Here's how the part is built. I have some questions about the finished solid (model axes, mm). Coordinates: 2 decimals unless noted, no trailing zeros. Write each loop counter-clockwise with the first axis right and the second up, starting at its lowest first coordinate (ties: lowest second). Pieces come first, ordered by that corner, then holes.
(1) Please list where these lines run through material, in increasing order: probe 1 along Y at (x, z) = (0, 2.9); probe 2 along Y at (x, z) = (-25.4, 1.1); probe 3 along Y at (x, z) = (30, 0.2).
(2) Imagine slicing it at B-B, the plane y = -56.65. List the corners of the cut face in (x, z) for me.
(3) Imagine slicing it at C-C, the plane z = 1.2. List the corners of the cut face in (x, y) for me, plus the area to 3 significant figures.
(4) Imagine slicing it at D-D, the plane y = -95.25. List the corners of the cut face in (x, z) for me, plus the area to 3 significant figures.
(5) Imagine slicing it at A-A, the plane x = 0. List the corners of the cut face in (y, z) for me, plus the area to 3 significant figures.
Autodesk Inventor part; units mm, degrees
ref_plane "Work Plane1" through (0, -135.7786, 0) normal (0, 0, 1) x (1, 0, 0)
ref_plane "YZ Plane" through (0, 0, 0) normal (1, 0, 0) x (0, 1, 0)
ref_plane "XZ Plane" through (0, 0, 0) normal (0, 1, 0) x (-1, 0, 0)
sketch "Sketch1" plane through (0, 0, 0) normal (0, 0, 1) x (1, 0, 0)
  line L0 (6.35, -214.55) -> (43.1, -214.55)
  line L1 (43.1, -214.55) -> (43.1, -189.15)
  line L2 (43.1, -189.15) -> (40.1028, -189.15)
  line L3 (40.1028, -189.15) -> (40.1028, -176.45)
  line L4 (40.1028, -176.45) -> (43.1, -176.45)
  line L5 (43.1, -176.45) -> (43.1, -110.25)
  line L6 (43.1, -110.25) -> (40.1028, -110.25)
  line L7 (40.1028, -110.25) -> (40.1028, -97.55)
  line L8 (40.1028, -97.55) -> (43.1, -97.55)
  line L9 (43.1, -97.55) -> (43.1, -72.15)
  line L10 (43.1, -72.15) -> (35.023, -72.15)
  arc A0 (-35.023, -72.15) -> (35.023, -72.15) centre (0, -57.15) ccw
  line L11 (-35.023, -72.15) -> (-43.1, -72.15)
  line L12 (-43.1, -72.15) -> (-43.1, -97.55)
  line L13 (-43.1, -97.55) -> (-40.1028, -97.55)
  line L14 (-40.1028, -97.55) -> (-40.1028, -110.25)
  line L15 (-40.1028, -110.25) -> (-43.1, -110.25)
  line L16 (-43.1, -110.25) -> (-43.1, -176.45)
  line L17 (-43.1, -176.45) -> (-40.1028, -176.45)
  line L18 (-40.1028, -176.45) -> (-40.1028, -189.15)
  line L19 (-40.1028, -189.15) -> (-43.1, -189.15)
  line L20 (-43.1, -189.15) -> (-43.1, -214.55)
  line L21 (-43.1, -214.55) -> (-6.35, -214.55)
  line L22 (-11.16, -143.04) -> (-11.16, -138.135)
  line L23 (-11.16, -138.135) -> (10.16, -138.135)
  line L24 (10.16, -138.135) -> (10.16, -168.265)
  line L25 (10.16, -168.265) -> (-11.16, -168.265)
  line L26 (-11.16, -168.265) -> (-11.16, -159.55)
  line L27 (-11.16, -159.55) -> (-19.058, -159.55)
  line L28 (-19.058, -159.55) -> (-19.058, -164.622)
  line L29 (-19.058, -164.622) -> (-22.598, -164.622)
  line L30 (-22.598, -164.622) -> (-22.598, -159.55)
  line L31 (-22.598, -159.55) -> (-32.258, -159.55)
  line L32 (-32.258, -159.55) -> (-32.258, -167.805)
  line L33 (-32.258, -167.805) -> (-34.29, -167.805)
  line L34 (-34.29, -167.805) -> (-34.29, -159.55)
  line L35 (-34.29, -159.55) -> (-38.1, -159.55)
  line L36 (-38.1, -159.55) -> (-38.1, -136.69)
  line L37 (-38.1, -136.69) -> (-22.598, -136.69)
  line L38 (-22.598, -136.69) -> (-22.598, -131.618)
  line L39 (-22.598, -131.618) -> (-19.058, -131.618)
  line L40 (-19.058, -131.618) -> (-19.058, -136.69)
  line L41 (-19.058, -136.69) -> (-15.24, -136.69)
  line L42 (-15.24, -136.69) -> (-15.24, -143.04)
  arc A1 (-38.1, -57.15) -> (38.1, -57.15) centre (0, -57.15) ccw
  line L43 (0, -57.15) -> (0, -82.55)
  circle A2 centre (0, -82.55) radius 38.1
  line L44 (38.1, -82.55) -> (-38.1, -82.55)
  line L45 (-38.1, -82.55) -> (-38.1, -44.45)
  line L46 (-38.1, -44.45) -> (38.1, -44.45)
  line L47 (38.1, -44.45) -> (38.1, -82.55)
  circle A3 centre (25.4, -95.25) radius 1.5
  circle A4 centre (-25.4, -95.25) radius 1.5
  line L48 (-15.24, -143.04) -> (-11.16, -143.04)
  line L49 (-6.35, -214.55) -> (-6.35, -203.8154)
  line L50 (-6.35, -203.8154) -> (6.35, -203.8154)
  line L51 (6.35, -203.8154) -> (6.35, -214.55)
  point P0 (0, 0)
  dimension "d1" = 76.2
  dimension "d0" = 25.4
extrude "Extrusion1" add sketch "Sketch1" along normal blind 4 contours L47 A2 L10 | L10 A2 A1 L47 | A2 L44 A0 L10 | L10 A1 A2 | A1 A2 L46 L47 | A2 L44 A0 | A0 L44 A1 A2 | L45 L11 A2 | A2 L11 A0 L44 | A0 L44 | A2 A1 L45 L46 | A2 A1 L11 | L11 L45 A1 A2 | A3 | A4
ref_plane "Work Plane1" through (0, -135.7786, 0) normal (0, 0, 1) x (1, 0, 0)
sketch "Sketch2" plane through (0, 0, 4) normal (0, 0, 1) x (1, 0, 0)
  line L0 (-40.1, -31.75) -> (-43.1, -31.75)
  line L1 (-43.1, -31.75) -> (-43.1, -57.15)
  line L2 (-43.1, -57.15) -> (-38.1, -57.15)
  arc A0 (-38.1, -57.15) -> (38.1, -57.15) centre (0, -57.15) ccw
  line L3 (38.1, -57.15) -> (43.1, -57.15)
  line L4 (43.1, -57.15) -> (43.1, -31.75)
  line L5 (43.1, -31.75) -> (40.1, -31.75)
  line L6 (40.1, -31.75) -> (40.1, -19.05)
  line L7 (40.1, -19.05) -> (43.1, -19.05)
  line L8 (43.1, -19.05) -> (43.1, 24.05)
  line L9 (43.1, 24.05) -> (40.1, 24.05)
  line L10 (40.1, 24.05) -> (40.1, 36.75)
  line L11 (40.1, 36.75) -> (43.1, 36.75)
  line L12 (43.1, 36.75) -> (43.1, 62.15)
  line L13 (14, 62.15) -> (-14, 62.15)
  line L14 (-43.1, 62.15) -> (-43.1, 36.75)
  line L15 (-43.1, 36.75) -> (-40.1, 36.75)
  line L16 (-40.1, 36.75) -> (-40.1, 24.05)
  line L17 (-40.1, 24.05) -> (-43.1, 24.05)
  line L18 (-43.1, 24.05) -> (-43.1, -19.05)
  line L19 (-43.1, -19.05) -> (-40.1, -19.05)
  line L20 (-40.1, -19.05) -> (-40.1, -31.75)
  line L21 (15.24, -5.55) -> (11.16, -5.55)
  line L22 (11.16, -5.55) -> (11.16, -14.265)
  line L23 (11.16, -14.265) -> (-10.16, -14.265)
  line L24 (-10.16, -14.265) -> (-10.16, 15.865)
  line L25 (-10.16, 15.865) -> (11.16, 15.865)
  line L26 (11.16, 15.865) -> (11.16, 7.15)
  line L27 (11.16, 7.15) -> (19.058, 7.15)
  line L28 (22.598, 7.15) -> (32.266, 7.15)
  line L29 (32.266, 7.15) -> (32.266, 15.405)
  line L30 (32.266, 15.405) -> (34.282, 15.405)
  line L31 (34.282, 15.405) -> (34.282, 7.15)
  line L32 (34.282, 7.15) -> (38.1, 7.15)
  line L33 (38.1, 7.15) -> (38.1, -15.71)
  line L34 (38.1, -15.71) -> (22.598, -15.71)
  line L35 (19.058, -15.71) -> (15.24, -15.71)
  line L36 (15.24, -15.71) -> (15.24, -5.55)
  line L37 (19.058, 7.15) -> (19.058, 12.222)
  line L38 (19.058, 12.222) -> (22.598, 12.222)
  line L39 (22.598, 12.222) -> (22.598, 7.15)
  line L40 (22.598, -15.71) -> (22.598, -20.782)
  line L41 (22.598, -20.782) -> (19.058, -20.782)
  line L42 (19.058, -20.782) -> (19.058, -15.71)
  line L43 (-14, 62.15) -> (-14, 31.5)
  line L44 (-14, 31.5) -> (-30.4, 31.5)
  line L45 (-30.4, 31.5) -> (-30.4, 62.15)
  line L46 (-30.4, 62.15) -> (-43.1, 62.15)
  line L47 (43.1, 62.15) -> (30.4, 62.15)
  line L48 (30.4, 62.15) -> (30.4, 31.5)
  line L49 (30.4, 31.5) -> (14, 31.5)
  line L50 (14, 31.5) -> (14, 62.15)
  line L51 (0, -57.15) -> (0, -56.65)
  circle A1 centre (0, -56.65) radius 2.5019
  point P0 (0, 0)
  dimension "d13" = 0.5
  dimension "d14" = 5.0038
extrude "Extrusion2" cut sketch "Sketch2" against normal blind 4 contours A1
sketch "Sketch3" plane through (0, 0, 4) normal (0, 0, 1) x (1, 0, 0)
  arc A0 (-35.023, -72.15) -> (35.023, -72.15) centre (0, -57.15) ccw
  line L0 (-6.35, -214.55) -> (-6.35, -203.8154)
  line L1 (-6.35, -203.8154) -> (6.35, -203.8154)
  line L2 (6.35, -203.8154) -> (6.35, -214.55)
  line L3 (6.35, -214.55) -> (43.1, -214.55)
  line L4 (43.1, -214.55) -> (43.1, -189.15)
  line L5 (43.1, -189.15) -> (40.1028, -189.15)
  line L6 (40.1028, -189.15) -> (40.1028, -176.45)
  line L7 (40.1028, -176.45) -> (43.1, -176.45)
  line L8 (43.1, -176.45) -> (43.1, -110.25)
  line L9 (43.1, -110.25) -> (40.1028, -110.25)
  line L10 (40.1028, -110.25) -> (40.1028, -97.55)
  line L11 (40.1028, -97.55) -> (43.1, -97.55)
  line L12 (43.1, -97.55) -> (43.1, -72.15)
  line L13 (43.1, -72.15) -> (35.023, -72.15)
  arc A1 (-35.023, -72.15) -> (35.023, -72.15) centre (0, -57.15) ccw
  line L14 (-35.023, -72.15) -> (-43.1, -72.15)
  line L15 (-43.1, -72.15) -> (-43.1, -97.55)
  line L16 (-43.1, -97.55) -> (-40.1028, -97.55)
  line L17 (-40.1028, -97.55) -> (-40.1028, -110.25)
  line L18 (-40.1028, -110.25) -> (-43.1, -110.25)
  line L19 (-43.1, -110.25) -> (-43.1, -176.45)
  line L20 (-43.1, -176.45) -> (-40.1028, -176.45)
  line L21 (-40.1028, -176.45) -> (-40.1028, -189.15)
  line L22 (-40.1028, -189.15) -> (-43.1, -189.15)
  line L23 (-43.1, -189.15) -> (-43.1, -214.55)
  line L24 (-43.1, -214.55) -> (-6.35, -214.55)
  line L25 (-11.16, -143.04) -> (-11.16, -138.135)
  line L26 (-11.16, -138.135) -> (10.16, -138.135)
  line L27 (10.16, -138.135) -> (10.16, -168.265)
  line L28 (10.16, -168.265) -> (-11.16, -168.265)
  line L29 (-11.16, -168.265) -> (-11.16, -159.55)
  line L30 (-11.16, -159.55) -> (-19.058, -159.55)
  line L31 (-19.058, -159.55) -> (-19.058, -164.622)
  line L32 (-19.058, -164.622) -> (-22.598, -164.622)
  line L33 (-22.598, -164.622) -> (-22.598, -159.55)
  line L34 (-22.598, -159.55) -> (-32.258, -159.55)
  line L35 (-32.258, -159.55) -> (-32.258, -167.805)
  line L36 (-32.258, -167.805) -> (-34.29, -167.805)
  line L37 (-34.29, -167.805) -> (-34.29, -159.55)
  line L38 (-34.29, -159.55) -> (-38.1, -159.55)
  line L39 (-38.1, -159.55) -> (-38.1, -136.69)
  line L40 (-38.1, -136.69) -> (-22.598, -136.69)
  line L41 (-22.598, -136.69) -> (-22.598, -131.618)
  line L42 (-22.598, -131.618) -> (-19.058, -131.618)
  line L43 (-19.058, -131.618) -> (-19.058, -136.69)
  line L44 (-19.058, -136.69) -> (-15.24, -136.69)
  line L45 (-15.24, -136.69) -> (-15.24, -143.04)
  arc A2 (-38.1, -82.55) -> (38.1, -82.55) centre (0, -82.55) ccw
  line L46 (38.1, -82.55) -> (38.1, -44.45)
  line L47 (38.1, -44.45) -> (-38.1, -44.45)
  line L48 (-38.1, -44.45) -> (-38.1, -82.55)
  line L49 (0, -95.25) -> (25.4, -95.25)
  line L50 (25.4, -95.25) -> (-25.4, -95.25)
  circle A3 centre (25.4, -95.25) radius 2
  circle A4 centre (-25.4, -95.25) radius 2
  circle A5 centre (25.4, -95.25) radius 1.5
  circle A6 centre (-25.4, -95.25) radius 1.5
  line L51 (-15.24, -143.04) -> (-11.16, -143.04)
  point P0 (0, 0)
  dimension "d7" = 25.4
  dimension "d8" = 50.8
  dimension "d9" = 4
  dimension "d10" = 4
extrude "Extrusion3" cut sketch "Sketch3" against normal blind 25.4 contours A3 | A4 | A5 | A6
properties part number "LargeConnectorBodies"
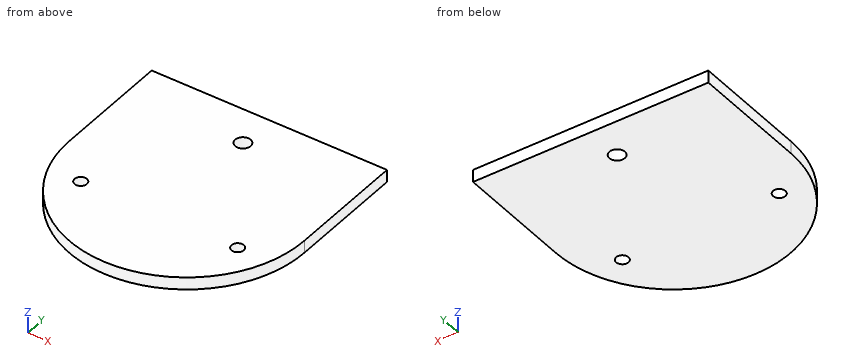
Recorded:
1. probe 1: y = -120.65 to -59.15, -54.15 to -44.45
1. probe 2: y = -110.95 to -97.25, -93.25 to -44.45
1. probe 3: y = -106.04 to -44.45
2. outline: (-38.1, 0) - (-2.5, 0) - (-2.5, 4) - (-38.1, 4) - close; (2.5, 0) - (38.1, 0) - (38.1, 4) - (2.5, 4) - close
3. outline: (-38.1, -82.55) arc R38.1 ccw to (38.1, -82.55) - (38.1, -44.45) - (-38.1, -44.45) - close; hole circle Ø4 at (-25.4, -95.25); hole circle Ø5 at (0, -56.65); hole circle Ø4 at (25.4, -95.25)
3. area: 5,140 mm2
4. outline: (-35.92, 0) - (-27.4, 0) - (-27.4, 4) - (-35.92, 4) - close; (-23.4, 0) - (23.4, 0) - (23.4, 4) - (-23.4, 4) - close; (27.4, 0) - (35.92, 0) - (35.92, 4) - (27.4, 4) - close
4. area: 255 mm2
5. outline: (-120.65, 0) - (-59.15, 0) - (-59.15, 4) - (-120.65, 4) - close; (-54.15, 0) - (-44.45, 0) - (-44.45, 4) - (-54.15, 4) - close
5. area: 285 mm2
